```python
from build123d import *

# Parameters (mm, degrees)
SKETCH1_W           = 96
SKETCH1_H           = 41
SKETCH1_W_2         = 80
SKETCH1_H_2         = 25
BOSS_EXTRUDE1_DEPTH = 10
FILLET1_R           = 3
SKETCH2_R           = 2
CUT_EXTRUDE1_DEPTH  = 99.672437894
SKETCH3_R           = 2.80429848
CUT_EXTRUDE5_DEPTH  = 64.914004725
FILLET2_R           = 3


with BuildPart() as part:
    # Sketch1 → Boss-Extrude1 (new body)
    with BuildSketch(Plane(origin=(0, 0, 0), x_dir=(1, 0, 0), z_dir=(0, 1, 0))):
        Rectangle(SKETCH1_W, SKETCH1_H)
        Rectangle(SKETCH1_W_2, SKETCH1_H_2, mode=Mode.SUBTRACT)
    extrude(amount=BOSS_EXTRUDE1_DEPTH)

    # Fillet1
    fillet1_edges = [part.edges().sort_by_distance(p)[0] for p in [
        (48, 5, 20.5),
        (-48, 5, 20.5),
        (-48, 5, -20.5),
        (48, 5, -20.5),
    ]]
    fillet(fillet1_edges, radius=FILLET1_R)

    # Sketch2 → Cut-Extrude1 (cut, through all)
    with BuildSketch(Plane.ZY.offset(48)):
        with Locations((0, 5)):
            Circle(SKETCH2_R)
    extrude(amount=-CUT_EXTRUDE1_DEPTH, mode=Mode.SUBTRACT)

    # Sketch3 → Cut-Extrude5 (cut, through all)
    with BuildSketch(Plane.XY.offset(20.5)):
        with Locations((-22.5, 5)):
            Circle(SKETCH3_R)
        with Locations((0, 5)):
            Circle(SKETCH3_R)
        with Locations((22.5, 5)):
            Circle(SKETCH3_R)
    extrude(amount=-CUT_EXTRUDE5_DEPTH, mode=Mode.SUBTRACT)

    # Fillet2
    fillet2_edges = [part.edges().sort_by_distance(p)[0] for p in [
        (40, 5, 12.5),
        (40, 5, -12.5),
        (-40, 5, -12.5),
        (-40, 5, 12.5),
    ]]
    fillet(fillet2_edges, radius=FILLET2_R)


solid = part.part
```
Part model, mm, in its own coordinate system. A direction names the side the tool comes from. Round coordinates to 2 decimals unless told otherwise and drop trailing zeros. Write each loop counter-clockwise with the first axis right and the second up, starting at its lowest first coordinate (ties: lowest second). Pieces come first, ordered by that corner, then holes. Notation, with made-up numbers: (88, -5.75) -> (96, -5.75) arc R14 ccw to (96, 10.25) -> close; hole circle Ø5 at (-18.5, 52). An arc over 180 degrees is marked (long way). Return JSON: item names as keys, results as strings. Group by question number.
Q1. Probe L1, parallel to X at y = 3.25, z = -6; L2, parallel to X at y = 4.5, z = 17.5; L3, parallel to Z at x = 8, y = 8.75. List the from-to ranges inside material, lowest first. Write a range as [from, to].
Q2. Saw through at B-B on x = -36. Write the cut outline in (y, z).
Q3. Saw through at A-A on z = 0. Write the cut outline in (x, y), plus the area to 3 significant figures.
Q4. Which spindle directions (+Z, -Z, +X, -X, +Y, -Y) get a long thin tool onto all of the face, cutting with end or side? Do faces 1 (the flat face through (-1, 2, -12.5)), 2 (the cylindrical face through (-44, 7, 0)). Say none if no direction does.
Q5. Saw through at D-D on y = 9. Write the cut outline in (x, z).
Q6. Saw through at C-C on z = -7. Write the cut outline in (x, y), plus the area to 3 significant figures.
Q7. Pin check, flat tip, straight feed: pin 1 (5 mm diameter, centred on x = 0, y = 5, fed in from -Z). Stop position of the tip, or through.
Q8. Mould opens along Z. For faces 3 (the cylindrical face through (20.275, 3.294, 16.556)), 4 (the cylindrical face through (47.1, 5.07, -19.64)), 5 (the cylindrical face through (-39.1, 5.07, -11.64)), 6 (the cylindrical face through (39.14, 5.07, -11.6)) say: pulls with the +Z half, pulls with the -Z half, needs draft (parallel to the pull), parting line crosses it, or undercut.
Answer:
{
 "1": {"L1": "[-48, -40], [40, 48]", "L2": "[-48, -25.26], [-19.74, -2.76], [2.76, 19.74], [25.26, 48]", "L3": "[-20.5, -12.5], [12.5, 20.5]"},
 "2": {"outline": "(0, -20.5) -> (10, -20.5) -> (10, -12.5) -> (0, -12.5) -> close; (0, 12.5) -> (10, 12.5) -> (10, 20.5) -> (0, 20.5) -> close"},
 "3": {"outline": "(-48, 0) -> (-40, 0) -> (-40, 3) -> (-48, 3) -> close; (-48, 7) -> (-40, 7) -> (-40, 10) -> (-48, 10) -> close; (40, 0) -> (48, 0) -> (48, 3) -> (40, 3) -> close; (40, 7) -> (48, 7) -> (48, 10) -> (40, 10) -> close", "area": "96.0 mm2"},
 "4": {"face 1": "+Y, -Y", "face 2": "+X, -X"},
 "5": {"outline": "(-48, -17.5) arc R3 ccw to (-45, -20.5) -> (45, -20.5) arc R3 ccw to (48, -17.5) -> (48, 17.5) arc R3 ccw to (45, 20.5) -> (-45, 20.5) arc R3 ccw to (-48, 17.5) -> close; hole (-40, -9.5) arc R3 ccw to (-37, -12.5) -> (37, -12.5) arc R3 ccw to (40, -9.5) -> (40, 9.5) arc R3 ccw to (37, 12.5) -> (-37, 12.5) arc R3 ccw to (-40, 9.5) -> close"},
 "6": {"outline": "(-48, 0) -> (-40, 0) -> (-40, 10) -> (-48, 10) -> close; (40, 0) -> (48, 0) -> (48, 10) -> (40, 10) -> close", "area": "160 mm2"},
 "7": {"pin 1": "through"},
 "8": {"face 3": "needs draft", "face 4": "pulls with the -Z half", "face 5": "undercut", "face 6": "undercut"}
}
